Geometry check sheet. Reference: the model listing, model coordinates, mm. Coordinates: 2 decimals unless noted, no trailing zeros. Order: outer loops, then holes, each group sorted by start corner. A loop starts at its lowest first (then second) coordinate and runs counter-clockwise, first axis right, second up. Notation, with made-up numbers: (-25, -6) - (5, -6) arc R33 cw to (5, 23) - close; hole circle Ø11 at (54, 34.25). An arc over 180 degrees is marked (long way). Return JSON: item names as keys, results as strings. Group by question number.
Item 1: Scan lines: probe 1 along X at (y, z) = (3, 15.5); probe 2 along X at (y, z) = (-0.5, 13); probe 3 along Y at (x, z) = (2.25, 14.5). Record each from-to range of solid material in increasing order.
Item 2: Section check A-A on x = 0. Enter the section's corners in (y, z).
Item 3: Section check D-D on z = 6.5. Enter the section's corners in (x, y).
Item 4: Gauge pin test, flat ends, axial feed: pin 1 (6 mm diameter, centred on x = -2.5, z = 14.5, fed in from +Y); pin 2 (6 mm diameter, centred on x = 3.5, z = 17, fed in from -Y). Record the tip position at first contact, or that the pin passes through.
Item 5: Section check C-C on z = 14.5. Enter the section's corners in (x, y), then the cut area to 3 significant figures.
from build123d import *

# Parameters (mm, degrees)
SKETCH_1_R      = 3.5
EXTRUDE_1_DEPTH = 22
FILLET_1_R      = 1
SKETCH_2_R      = 5
EXTRUDE_2_DEPTH = 14
CHAMFER_1_SIZE  = 2


# Read off the part's stored shape, not the designer's step: M10 机械螺纹 螺柱1
with BuildPart() as part:
    # 草图1 → 凸台-拉伸1 (new body)
    with BuildSketch(Plane.XY):
        Circle(SKETCH_1_R)
    extrude(amount=EXTRUDE_1_DEPTH)

    # 圆角1
    fillet_1_edges = [part.edges().sort_by_distance(p)[0] for p in [
        (-3.5, 0, 22),
    ]]
    fillet(fillet_1_edges, radius=FILLET_1_R)

    # 草图2 → 凸台-拉伸2 (add)
    with BuildSketch(Plane(origin=(0, 0, 0), x_dir=(-1, 0, 0), z_dir=(0, 0, -1))):
        Circle(SKETCH_2_R)
    extrude(amount=-EXTRUDE_2_DEPTH)

    # M10 机械螺纹 螺柱1 outline → M10 机械螺纹 螺柱1 (revolve, cut)
    with BuildSketch(Plane.XZ):
        Polygon((5, 0.812), (4.188, 0), (5, 0), align=None)
    revolve(axis=Axis((0, 0, 0), (0, 0, 1)), mode=Mode.SUBTRACT)

    # 倒角1
    # the kernel refuses this chamfer: 2 mm, written as the material it takes off along each edge
    with BuildSketch(Plane(origin=(0, 0, 14), x_dir=(-1, 0, 0), z_dir=(0, -1, 0))) as chamfer_1_piece_1_section:
        Polygon((5, CHAMFER_1_SIZE), (5 - CHAMFER_1_SIZE, 0), (5, 0), align=None)
    chamfer_1_piece_1 = revolve(axis=Axis((0, 0, 14), (0, 0, -1)), mode=Mode.PRIVATE)
    chamfer_1_piece_1 = chamfer_1_piece_1 - Plane(origin=(0, 0, 12.748861674), x_dir=(1, 0, 0), z_dir=(0, 0, -1)) * Cylinder(3.5, 20, mode=Mode.PRIVATE)
    add(chamfer_1_piece_1, mode=Mode.SUBTRACT)


solid = part.part
Computed:
{
 "1": {"probe 1": "x = -1.8 to 1.8", "probe 2": "x = -3.97 to 3.97", "probe 3": "y = -2.68 to 2.68"},
 "2": {"outline": "(-5, 0.81) - (-4.19, 0) - (4.19, 0) - (5, 0.81) - (5, 12) - (3.5, 13.5) - (3.5, 21) arc R1 ccw to (2.5, 22) - (-2.5, 22) arc R1 ccw to (-3.5, 21) - (-3.5, 13.5) - (-5, 12) - close"},
 "3": {"outline": "circle Ø10 at (0, 0)"},
 "4": {"pin 1": "stops at y = 4.93", "pin 2": "stops at y = -3.46"},
 "5": {"outline": "circle Ø7 at (0, 0)", "area": "38.5 mm²"}
}
